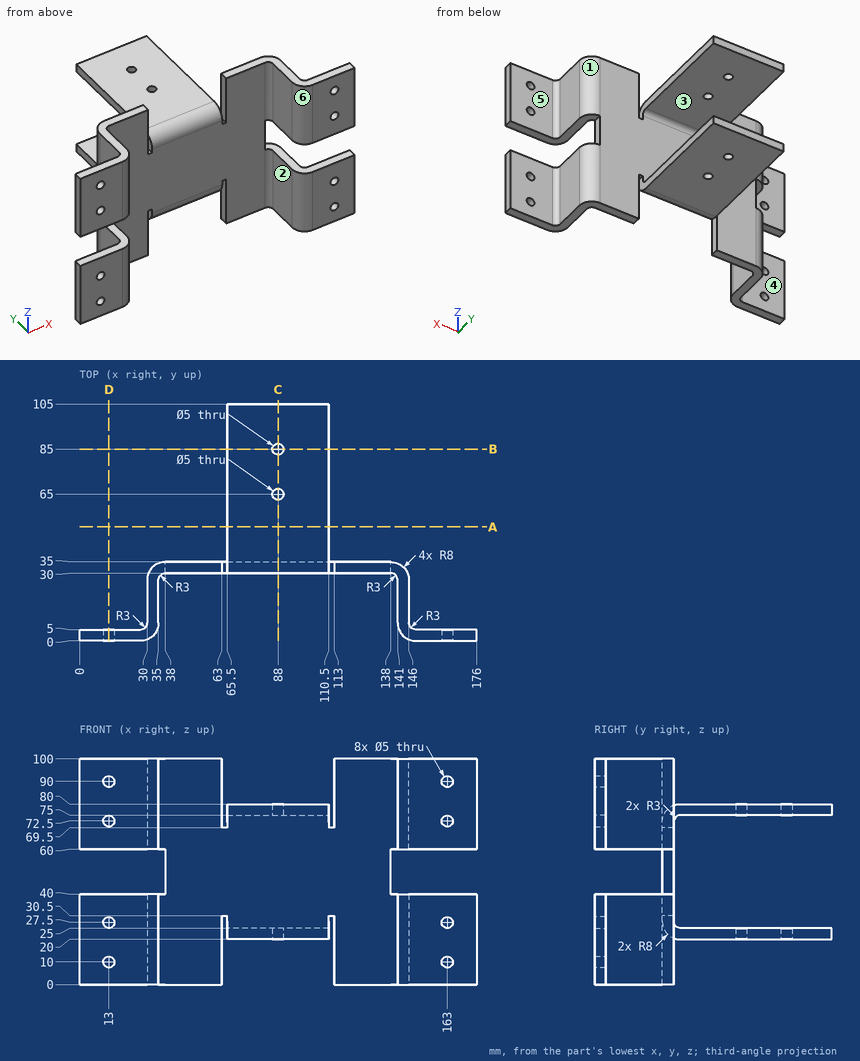
Check sheet for the drawn part. Datum: minimum x, y, z corner. Units: mm. A direction names the side the tool comes from. Coordinates: 2 decimals unless noted, no trailing zeros. Order: outer loops, then holes, each group sorted by start corner. A loop starts at its lowest first (then second) coordinate and runs counter-clockwise, first axis right, second up. Notation, with made-up numbers: (87, 67) -> (131, 67) arc R22 ccw to (131, 105) -> close; hole circle Ø3 at (15, 38). An arc over 180 degrees is marked (long way). Use a Markdown table: item, result. Add a question column.
1. Cross-section at B-B (y = 85). Enter the section's corners in (x, z).
2. Mould release check, pull along X, two halves, no side actions. Record for the marked faces 1, 2 and 3: pulls with the +X half, pulls with the -X half, needs draft (parallel to the pull), parting line crosses it, or undercut.
3. Material ranges on L1, parallel to Z at x = 163, y = 3; L2, parallel to Y at x = 88, z = 78.9; L3, parallel to X at y = 2, z = 10, recorded low to high.
4. Cross-section at A-A (y = 50.5). Enter the section's corners in (x, z), and give its area (3 significant figures).
5. Set-up check for the marked faces 4, 5 and 6: record each of +Z, -Z, +X, -X, +Y, -Y from which the full face is reachable in a straight line by a thin tool's end or side.
6. Cross-section at C-C (x = 88). Enter the section's corners in (y, z).
7. Cross-section at D-D (x = 13). Enter the section's corners in (y, z), and give its area (3 significant figures).
8. Go/stop test with flat-tipped pins: pin 1 Ø21 at (y, z) = (17.5, 25) entering from -X; pin 2 Ø1.2 at (x, y) = (111.5, 33) entering from -Z; pin 3 Ø17.5 at (x, y) = (160.5, 19) entering from +Z; pin 4 Ø9.5 at (y, z) = (15, 15) entering from -X. Record where each tip stops, or that it passes through.
Filled sheet:
| question | item | result |
|---|---|---|
| 1 | outline | (65.5, 20) -> (85.5, 20) -> (85.5, 25) -> (65.5, 25) -> close; (65.5, 75) -> (85.5, 75) -> (85.5, 80) -> (65.5, 80) -> close; (90.5, 20) -> (110.5, 20) -> (110.5, 25) -> (90.5, 25) -> close; (90.5, 75) -> (110.5, 75) -> (110.5, 80) -> (90.5, 80) -> close |
| 2 | face 1 | pulls with the +X half |
| 2 | face 2 | undercut |
| 2 | face 3 | needs draft |
| 3 | L1 | 0 to 7.5, 12.5 to 25, 30 to 40, 60 to 70, 75 to 87.5, 92.5 to 100 |
| 3 | L2 | 33.95 to 62.5, 67.5 to 82.5, 87.5 to 105 |
| 3 | L3 | 0 to 10.5, 15.5 to 32.29, 143.71 to 160.5, 165.5 to 176 |
| 4 | outline | (65.5, 20) -> (110.5, 20) -> (110.5, 25) -> (65.5, 25) -> close; (65.5, 75) -> (110.5, 75) -> (110.5, 80) -> (65.5, 80) -> close |
| 4 | area | 450 mm2 |
| 5 | face 4 | +Z, -Z, -X, +Y |
| 5 | face 5 | +Z, -Z, +X, +Y |
| 5 | face 6 | +Z, -Z, -Y |
| 6 | outline | (30, 28) arc R8 ccw to (38, 20) -> (62.5, 20) -> (62.5, 25) -> (38, 25) arc R3 cw to (35, 28) -> (35, 72) arc R3 cw to (38, 75) -> (62.5, 75) -> (62.5, 80) -> (38, 80) arc R8 ccw to (30, 72) -> close; (67.5, 20) -> (82.5, 20) -> (82.5, 25) -> (67.5, 25) -> close; (67.5, 75) -> (82.5, 75) -> (82.5, 80) -> (67.5, 80) -> close; (87.5, 20) -> (105, 20) -> (105, 25) -> (87.5, 25) -> close; (87.5, 75) -> (105, 75) -> (105, 80) -> (87.5, 80) -> close |
| 7 | outline | (0, 0) -> (5, 0) -> (5, 7.5) -> (0, 7.5) -> close; (0, 12.5) -> (5, 12.5) -> (5, 25) -> (0, 25) -> close; (0, 30) -> (5, 30) -> (5, 40) -> (0, 40) -> close; (0, 60) -> (5, 60) -> (5, 70) -> (0, 70) -> close; (0, 75) -> (5, 75) -> (5, 87.5) -> (0, 87.5) -> close; (0, 92.5) -> (5, 92.5) -> (5, 100) -> (0, 100) -> close |
| 7 | area | 300 mm2 |
| 8 | pin 1 | x = 29.83 |
| 8 | pin 2 | z = 30.5 |
| 8 | pin 3 | through |
| 8 | pin 4 | x = 30 |
